Part model, mm, in its own coordinate system. A direction names the side the tool comes from. Give positions to 0.01 mm unless a question says otherwise; leave off trailing zeros. Write each loop counter-clockwise with the first axis right and the second up, starting at its lowest first coordinate (ties: lowest second). Pieces come first, ordered by that corner, then holes. Notation, with made-up numbers: M 53.5,53.25 L 104.5,53.25 A24 ccw 104.5,88.25 Z; hole C 81.25,3.5 d3. An arc over 180 degrees is marked long. Use a Markdown table: item, result. Add a question column.
from build123d import *

# Parameters (mm, degrees)
SKETCH_R        = 73
SKETCH_R_2      = 1.75
PAD_DEPTH       = 3
SKETCH001_R     = 1.75
POCKET_DEPTH    = 415.994947
SKETCH002_R     = 1.75
POCKET001_DEPTH = 3.001
POCKET002_DEPTH = 3.001
SKETCH004_R     = 1.75
SKETCH004_R_2   = 1.5
POCKET003_DEPTH = 3.001


with BuildPart() as part:
    # Sketch → Pad (new body)
    with BuildSketch(Plane.XY):
        Circle(SKETCH_R)
        with Locations((-15, 49)):
            Circle(SKETCH_R_2, mode=Mode.SUBTRACT)
        with Locations((15, 49)):
            Circle(SKETCH_R_2, mode=Mode.SUBTRACT)
        with Locations((15, 25)):
            Circle(SKETCH_R_2, mode=Mode.SUBTRACT)
        with Locations((-15, 25)):
            Circle(SKETCH_R_2, mode=Mode.SUBTRACT)
    extrude(amount=PAD_DEPTH)

    # Sketch001 (on Face7 of Pad) → Pocket (cut, through all)
    with BuildSketch(Plane.XY.offset(3)):
        with Locations((-45.5, -5)):
            Circle(SKETCH001_R)
        with Locations((-36.5, -5)):
            Circle(SKETCH001_R)
        with Locations((-45.5, -40)):
            Circle(SKETCH001_R)
        with Locations((-36.5, -40)):
            Circle(SKETCH001_R)
        with Locations((-10, -22.5)):
            Circle(SKETCH001_R)
        with BuildLine():
            Line((-77, 2.5), (-58.5, 2.5))
            ThreePointArc((-57, 1), (-57.43934, 2.06066), (-58.5, 2.5))
            Line((-57, 1), (-57, -47.5))
            Line((-57, -47.5), (-77, -47.5))
            Line((-77, -47.5), (-77, 2.5))
        make_face()
    pocket = extrude(amount=-POCKET_DEPTH, mode=Mode.SUBTRACT)

    # Mirrored: Pocket across YZ
    add(pocket.mirror(Plane.YZ), mode=Mode.SUBTRACT)

    # Sketch002 (on Face4 of Mirrored) → Pocket001 (cut, through all)
    with BuildSketch(Plane.XY.offset(3)):
        with Locations((-40, -52.497619)):
            Circle(SKETCH002_R)
        with Locations((40, -52.497619)):
            Circle(SKETCH002_R)
        with Locations((-50, 43.081318)):
            Circle(SKETCH002_R)
        with Locations((50, 43.081318)):
            Circle(SKETCH002_R)
    extrude(amount=-POCKET001_DEPTH, mode=Mode.SUBTRACT)

    # Sketch003 (on Face4 of Pocket001) → Pocket002 (cut, through all)
    with BuildSketch(Plane.XY.offset(3)):
        with BuildLine():
            ThreePointArc((-48, 7), (-51.5, 3.5), (-48, 0))
            Line((-48, 0), (-34, 0))
            ThreePointArc((-34, 0), (-30.5, 3.5), (-34, 7))
            Line((-48, 7), (-34, 7))
        make_face()
        with BuildLine():
            ThreePointArc((34, 7), (30.5, 3.5), (34, 0))
            Line((34, 0), (48, 0))
            ThreePointArc((48, 0), (51.5, 3.5), (48, 7))
            Line((34, 7), (48, 7))
        make_face()
    extrude(amount=-POCKET002_DEPTH, mode=Mode.SUBTRACT)

    # Sketch004 (on Face4 of Pocket002) → Pocket003 (cut, through all)
    with BuildSketch(Plane.XY.offset(3)):
        with Locations((-12.5, -57)):
            Circle(SKETCH004_R)
        with Locations((12.5, -57)):
            Circle(SKETCH004_R)
        with Locations((-24.5, 59.56346)):
            Circle(SKETCH004_R_2)
        with Locations((24.5, 59.56346)):
            Circle(SKETCH004_R_2)
        with Locations((-24.5, 1.56346)):
            Circle(SKETCH004_R_2)
        with Locations((24.5, 1.56346)):
            Circle(SKETCH004_R_2)
        with Locations((-10, -35)):
            Circle(SKETCH004_R)
        with Locations((10, -35)):
            Circle(SKETCH004_R)
    extrude(amount=-POCKET003_DEPTH, mode=Mode.SUBTRACT)


solid = part.part
1. Cut at B-B (y = -57). Write the cut outline in (x, z), then the cut area to 3 significant figures.
2. Tool access for faces 5 (the cylindrical face through (-30.5, 3.4, 1.5)), 6 (the cylindrical face through (1.57, 72.983, 1.479)): list every direction of +Z, -Z, +X, -X, +Y, -Y with a clear straight run to the whole face (end or side of a thin tool).
3. Cut at A-A (y = 25). Write the cut outline in (x, z), then the cut area to 3 significant figures.
4. Flat gauge pins, fed straight in: pin 1 (0.9 mm diameter, centred on x = -37.5, z = 2, fed in from +Y); pin 2 (4.5 mm diameter, centred on x = -10, y = -22.5, fed in from -Z); pin 3 (0.9 mm diameter, centred on x = -69, z = 2, fed in from -Y); pin 4 (1.5 mm diameter, centred on x = 38, z = 1.5, fed in from -Y). Where does each tip first touch, or does it go through?
5. Mould opens along X. For faces 1 (the cylindrical face through (-0.916, -72.994, 1.479)), 2 (the cylindrical face through (10.228, -20.765, 1.521)), 3 (the flat face through (-1, 1, 0)), 4 (the cylindrical face through (11.669, -34.474, 1.521)) say: released by +X, released by -X, zero draft, split by the parting line, or undercut.
6. Cut at C-C (z = 1.7). Give the number of separate pieces and of enclosed holes in the cut face, then the cut area to 3 significant figures.
7. Drill centre lines: probe 1 along Y at (x, z) = (36.5, 2.2); probe 2 along Y at (x, z) = (-38.5, 0.7); probe 3 along Y at (x, z) = (41.5, 2.8). Where is each one in solid material? Low to high. Write a range as [from, to].
A:
| question | item | result |
|---|---|---|
| 1 | outline | M -45.61,0 L -14.25,0 L -14.25,3 L -45.61,3 Z; M -10.75,0 L 10.75,0 L 10.75,3 L -10.75,3 Z; M 14.25,0 L 45.61,0 L 45.61,3 L 14.25,3 Z |
| 1 | area | 253 mm² |
| 2 | face 5 | +Z, -Z |
| 2 | face 6 | +Z, -Z, +Y |
| 3 | outline | M -68.59,0 L -16.75,0 L -16.75,3 L -68.59,3 Z; M -13.25,0 L 13.25,0 L 13.25,3 L -13.25,3 Z; M 16.75,0 L 68.59,0 L 68.59,3 L 16.75,3 Z |
| 3 | area | 391 mm² |
| 4 | pin 1 | stops at y = 62.9 |
| 4 | pin 2 | stops at z = 0 |
| 4 | pin 3 | stops at y = 2.5 |
| 4 | pin 4 | stops at y = -62.78 |
| 5 | face 1 | split by the parting line |
| 5 | face 2 | undercut |
| 5 | face 3 | zero draft |
| 5 | face 4 | undercut |
| 6 | separate pieces | 1 |
| 6 | enclosed holes | 28 |
| 6 | area | 15,200 mm² |
| 7 | probe 1 | y = [-63.22, -41.75], [-38.25, -6.75], [-3.25, 0], [7, 63.22] |
| 7 | probe 2 | y = [-62.02, -53.4], [-51.6, 0], [7, 62.02] |
| 7 | probe 3 | y = [-60.06, -53.4], [-51.6, 0], [7, 60.06] |
